```python
from build123d import *

# Parameters (mm, degrees)
F1_DEPTH = 1996
F3_W     = 4
F3_H     = 87
F4_DEPTH = 21.409
F6_DEPTH = 4.001


with BuildPart() as f1:
    # F0 (on Front) → F1 (new body)
    with BuildSketch(Plane.XZ):
        with BuildLine():
            Line((-46.25, 34), (-46.25, -42))
            Line((-46.25, -42), (-42.25, -42))
            Line((-42.25, -42), (-42.25, 34))
            ThreePointArc((-42.25, 34), (-41.0784271247, 36.8284271247), (-38.25, 38))
            Line((-38.25, 38), (38.25, 38))
            ThreePointArc((38.25, 38), (41.0784271247, 36.8284271247), (42.25, 34))
            Line((42.25, 34), (42.25, -42))
            Line((42.25, -42), (46.25, -42))
            Line((46.25, -42), (46.25, 34))
            ThreePointArc((46.25, 34), (43.9068542495, 39.6568542495), (38.25, 42))
            Line((38.25, 42), (-38.25, 42))
            ThreePointArc((-38.25, 42), (-43.9068542495, 39.6568542495), (-46.25, 34))
        make_face()
    extrude(amount=-F1_DEPTH)

    # F3 (on face) → F4 (cut)
    with BuildSketch(Plane(origin=(-46.25, 0, 0), x_dir=(0, -1, 0), z_dir=(-1, 0, 0))):
        with Locations((-2, 0.3707238951)):
            Rectangle(F3_W, F3_H)
    extrude(amount=-F4_DEPTH, mode=Mode.SUBTRACT)

    # F5 (on face) → F6 (cut, through all)
    with BuildSketch(Plane(origin=(0, 0, 38), x_dir=(1, 0, 0), z_dir=(0, 0, -1))):
        with BuildLine():
            ThreePointArc((-19.7495876579, -14.5), (-21.0676071426, -11.3180194847), (-24.2495876579, -10))
            ThreePointArc((-24.2495876579, -10), (-28.7495876579, -14.5), (-24.2495876579, -19))
            ThreePointArc((-24.2495876579, -19), (-21.0676071426, -17.6819805153), (-19.7495876579, -14.5))
        make_face()
        with BuildLine():
            ThreePointArc((11.2504123421, -45.5), (9.9323928574, -42.3180194847), (6.7504123421, -41))
            ThreePointArc((6.7504123421, -41), (3.5684318267, -42.3180194847), (2.2504123421, -45.5))
            ThreePointArc((2.2504123421, -45.5), (6.7504123421, -50), (11.2504123421, -45.5))
        make_face()
    extrude(amount=-F6_DEPTH, mode=Mode.SUBTRACT)


solid = f1.part
```
Geometry check sheet. Reference: the model listing, model coordinates, mm. A direction names the side the tool comes from. Coordinates: 2 decimals unless noted, no trailing zeros. Order: outer loops, then holes, each group sorted by start corner. A loop starts at its lowest first (then second) coordinate and runs counter-clockwise, first axis right, second up. Notation, with made-up numbers: (-31, 58.25) - (15, 58.25) arc R21 cw to (15, 91.25) - close; hole circle Ø10 at (32, 61.5). An arc over 180 degrees is marked (long way). Use one line per item in the form item = value.
1. Gauge pin test, flat ends, axial feed: pin 1 (1.5 mm diameter, centred on x = -8.5, y = 1159, fed in from -Z); pin 2 (4.5 mm diameter, centred on y = 1, z = 41, fed in from -X). Record the tip position at first contact, or that the pin passes through.
Here are the results:
pin_1 = 38
pin_2 = -24.84
2. Section check A-A (z = -26). Record the boundary of the cut face in (x, y), then the cut area to 3 significant figures.
Here are the results:
outline = (-46.25, 4) - (-42.25, 4) - (-42.25, 1996) - (-46.25, 1996) - close; (42.25, 0) - (46.25, 0) - (46.25, 1996) - (42.25, 1996) - close
area = 16,000 mm²
3. Scan lines: line 1 (X direction, y = 1223, z = 34); line 2 (Z direction, x = 27, y = 608). Record each from-to range of solid material in increasing order.
Here are the results:
line_1 = -46.25 to -42.25, 42.25 to 46.25
line_2 = 38 to 42
4. Draft check along X on faces 1 (the face through (46.25, 984, -5)), 2 (the face through (-46.25, 986, -3)), 3 (the face through (42.25, 984, -3)). Enter one of: pulls with the +X half, pulls with the -X half, needs draft (parallel to the pull), parting line crosses it, or undercut.
Here are the results:
face_1 = pulls with the +X half
face_2 = pulls with the -X half
face_3 = undercut
5. Access from +Z, -Z, +X, -X, +Y, -Y to the whole of each face (thin tool, end or side, straight path). Record for faces 4 (the face through (45, 0, 19)), 5 (the face through (-42.25, 986, -5)).
Here are the results:
face_4 = +Z, -Z, +X, -X, -Y
face_5 = -Z, +Y, -Y
6. Section check B-B (y = 1339). Record the boundary of the cut face in (x, z).
Here are the results:
outline = (-46.25, -42) - (-42.25, -42) - (-42.25, 34) arc R4 cw to (-38.25, 38) - (38.25, 38) arc R4 cw to (42.25, 34) - (42.25, -42) - (46.25, -42) - (46.25, 34) arc R8 ccw to (38.25, 42) - (-38.25, 42) arc R8 ccw to (-46.25, 34) - close
